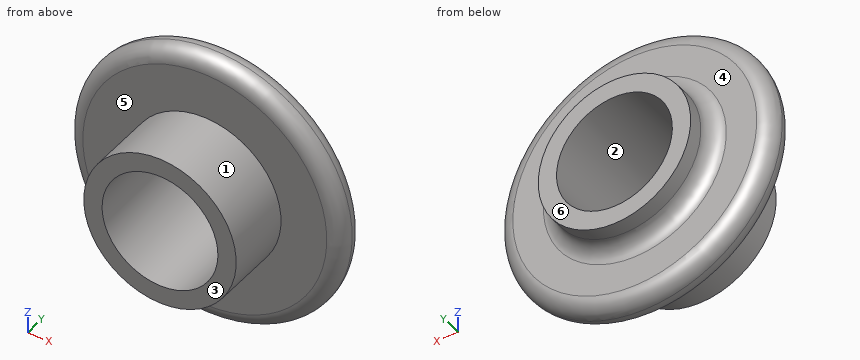
from build123d import *

# Parameters (mm, degrees)
FILLET1_R = 5


with BuildPart() as part:
    # Sketch1 → Revolve1 (revolve)
    with BuildSketch(Plane.XY, mode=Mode.PRIVATE) as revolve1_sk:
        Polygon((19, 0), (19, 42), (25, 42), (25, 32), (45, 32), (45, 22), (25, 22), (25, 0), align=None)
    revolve(revolve1_sk.sketch.rotate(Axis((0, 0, 0), (0, 1, 0)), 90), axis=Axis((0, 0, 0), (0, 1, 0)))

    # Fillet1
    fillet1_edges = [part.edges().sort_by_distance(p)[0] for p in [
        (0, 22, 45),
        (0, 32, 45),
        (0, 32, 25),
    ]]
    fillet(fillet1_edges, radius=FILLET1_R - 0.0001)  # a hair under: the kernel refuses the full size


solid = part.part
The listing builds one solid part. Answer for the finished solid, in the listing's coordinates (mm). Face numbers are marked on the shaded views. A direction names the side the tool comes from. Coordinates: 2 decimals unless noted, no trailing zeros. Order: outer loops, then holes, each group sorted by start corner. A loop starts at its lowest first (then second) coordinate and runs counter-clockwise, first axis right, second up. Notation, with made-up numbers: (-12.5, 53) -> (6.5, 53) arc R22 cw to (6.5, 68) -> close; hole circle Ø6 at (1, 67). An arc over 180 degrees is marked (long way). Answer in a Markdown table with one row per item. Add a question column.
Item 1: Determine the mould class of the marked faces 1, 2 and 3 for opening direction Z: +Z half, -Z half, draft (parallel to the pull), parting line (faces both ways), or undercut.
Item 2: Find section C-C (y = 7). Write down the section's boundary in (x, z), then the cut area to 3 significant figures.
Item 3: Each of these flat-tipped pins is pushed along its axis until it touches: P1, Ø1.5, axis at x = -2, y = 24, coming from the +Z side; P2, Ø2, axis at x = -5.5, y = 6, coming from the -Z side; P3, Ø3, axis at x = 9.5, z = -31.5, coming from the +Y side; P4, Ø24, axis at x = 1, z = 14.5, coming from the +Y side. Where does it stop, or does it pass through?
Item 4: Which of the six approach directions +Z, -Z, +X, -X, +Y, -Y give full straight-line access (tool end or side, diameter ignored) to the marked faces 4, 5 and 6?
Item 5: Find section D-D (y = 29.5). Write down the section's boundary in (x, z), then the cut area to 3 significant figures.
Item 6: Find the intervals of material crossed by L1, parallel to X at y = 16, z = 0; L2, parallel to Z at x = -0.5, y = 14 (3 decimals); L3, parallel to X at y = 28.5, z = -8.5, in increasing order. Write a range as from..to.
Result set:
| question | item | result |
|---|---|---|
| 1 | face 1 | parting line |
| 1 | face 2 | undercut |
| 1 | face 3 | draft |
| 2 | outline | circle Ø50 at (0, 0); hole circle Ø38 at (0, 0) |
| 2 | area | 829 mm² |
| 3 | P1 | stops at z = 44.42 |
| 3 | P2 | stops at z = -24.59 |
| 3 | P3 | stops at y = 32 |
| 3 | P4 | stops at y = 42 |
| 4 | face 4 | +Y |
| 4 | face 5 | -Y |
| 4 | face 6 | +Z, -Z, +X, -X, +Y |
| 5 | outline | circle Ø88.66 at (0, 0); hole circle Ø38 at (0, 0) |
| 5 | area | 5,040 mm² |
| 6 | L1 | x = -25..-19, 19..25 |
| 6 | L2 | z = -24.995..-18.993, 18.993..24.995 |
| 6 | L3 | x = -43.96..-16.99, 16.99..43.96 |
